from build123d import *

# Parameters (mm, degrees)
SKETCH1_R           = 27.5
BOSS_EXTRUDE1_DEPTH = 180
SKETCH2_R           = 27.5
BOSS_EXTRUDE2_DEPTH = 180
SKETCH3_R           = 27.5
BOSS_EXTRUDE3_DEPTH = 180


with BuildPart() as part:
    # Sketch1 → Boss-Extrude1 (new body)
    with BuildSketch(Plane.XY):
        with Locations(Location((0, 0, 0), (0, 0, 180))):
            Circle(SKETCH1_R)
    extrude(amount=BOSS_EXTRUDE1_DEPTH)

    # Sketch2 → Boss-Extrude2 (add)
    with BuildSketch(Plane.XY):
        with Locations(Location((0, 0, 0), (0, 0, 180))):
            Circle(SKETCH2_R)
    extrude(amount=BOSS_EXTRUDE2_DEPTH)

    # Sketch3 → Boss-Extrude3 (add)
    with BuildSketch(Plane.XY):
        with Locations(Location((0, 0, 0), (0, 0, 180))):
            Circle(SKETCH3_R)
    extrude(amount=BOSS_EXTRUDE3_DEPTH)


solid = part.part
Work out the finished part from the listing and answer in its coordinate system (mm). Round coordinates to 2 decimals unless told otherwise and drop trailing zeros. Write each loop counter-clockwise with the first axis right and the second up, starting at its lowest first coordinate (ties: lowest second). Pieces come first, ordered by that corner, then holes. Notation, with made-up numbers: M -25,85.5 L -6,85.5 A8 cw -6,90.5 Z; hole C 2,-10 d10. An arc over 180 degrees is marked long. Use a Markdown table: item, result.
1) The part is cut by section B-B on y = 20. Give the vertices of the cut face in (x, z), plus the area to 3 significant figures.
Taken from the geometry:
| item | result |
|---|---|
| outline | M -18.87,0 L 18.87,0 L 18.87,180 L -18.87,180 Z |
| area | 6,790 mm2 |
2) The part is cut by section C-C on x = 6. Give the vertices of the cut face in (y, z), plus the area to 3 significant figures.
Taken from the geometry:
| item | result |
|---|---|
| outline | M -26.84,0 L 26.84,0 L 26.84,180 L -26.84,180 Z |
| area | 9,660 mm2 |
3) Flat-ended cylindrical pins translate along their axes: pin 1 (8 mm diameter, centred on x = -5, z = 127.5, fed in from +Y); pin 2 (1.5 mm diameter, centred on y = -3.5, z = 67.5, fed in from +X); pin 3 (2 mm diameter, centred on x = 18, z = 116, fed in from -Y). Find the tip coordinate at first contact, or state that the pin passes through.
Taken from the geometry:
| item | result |
|---|---|
| pin 1 | stops at y = 27.48 |
| pin 2 | stops at x = 27.36 |
| pin 3 | stops at y = -21.62 |
4) Consider line 1 (Y direction, x = 15, z = 144); line 2 (X direction, y = 13.5, z = 37); line 3 (Y direction, x = -10, z = 25.5). Determine where each line is inside the solid, lowest interval first. Write a range as [from, to].
Taken from the geometry:
| item | result |
|---|---|
| line 1 | y = [-23.05, 23.05] |
| line 2 | x = [-23.96, 23.96] |
| line 3 | y = [-25.62, 25.62] |
5) The part is cut by section A-A on z = 149. Give the vertices of the cut face in (x, y).
Taken from the geometry:
| item | result |
|---|---|
| outline | C 0,0 d55 |
